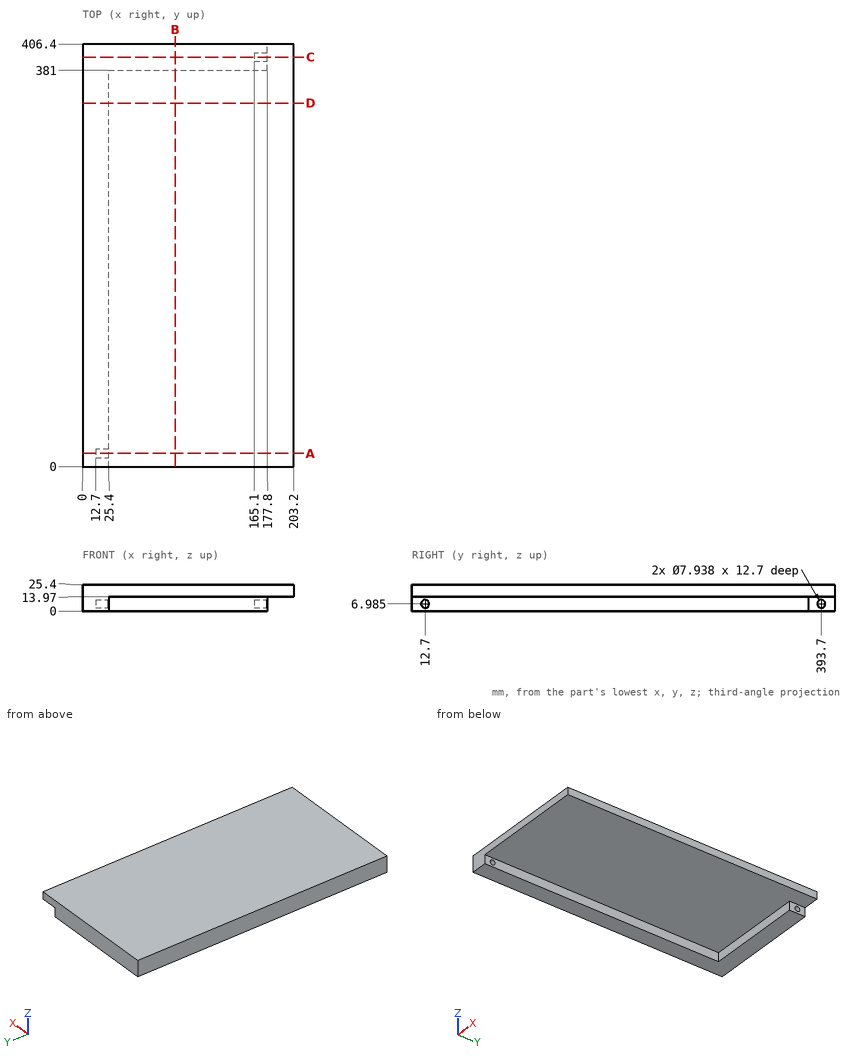
Geometry check sheet. Reference: drawing and pictorial views, mm from the part's lowest x, y, z. Coordinates: 2 decimals unless noted, no trailing zeros. Loops run counter-clockwise (first coordinate to the right, second up) from the corner with the lowest first, then second, coordinate; pieces in that order, holes last. Notation, with made-up numbers: (63, 3) -> (77, 3) arc R15 ccw to (77, 21) -> close; hole circle Ø10 at (12, 87). An arc over 180 degrees is marked (long way). Put each result on its own line as item: value.
1) Cross-section at D-D on y = 349.5. Record the boundary of the cut face in (x, z), plus the area to 3 significant figures.
Result set:
outline: (0, 0) -> (25.4, 0) -> (25.4, 13.97) -> (203.2, 13.97) -> (203.2, 25.4) -> (0, 25.4) -> close
area: 2,680 mm^2
2) Cross-section at A-A on y = 12.7. Record the boundary of the cut face in (x, z), plus the area to 3 significant figures.
Result set:
outline: (0, 0) -> (25.4, 0) -> (25.4, 3.02) -> (12.7, 3.02) -> (12.7, 10.95) -> (25.4, 10.95) -> (25.4, 13.97) -> (203.2, 13.97) -> (203.2, 25.4) -> (0, 25.4) -> close
area: 2,580 mm^2
3) Cross-section at B-B on x = 89. Record the boundary of the cut face in (y, z).
Result set:
outline: (0, 13.97) -> (381, 13.97) -> (381, 0) -> (406.4, 0) -> (406.4, 25.4) -> (0, 25.4) -> close
4) Cross-section at C-C on y = 393.7. Record the boundary of the cut face in (x, z).
Result set:
outline: (0, 0) -> (177.8, 0) -> (177.8, 3.02) -> (165.1, 3.02) -> (165.1, 10.95) -> (177.8, 10.95) -> (177.8, 13.97) -> (203.2, 13.97) -> (203.2, 25.4) -> (0, 25.4) -> close
5) Thickness scan on line 1 (Z direction, x = 19, y = 12.7); line 2 (Z direction, x = 20, y = 12); line 3 (Y direction, x = 99, z = 13). Record the ranges inside material, lowest first.
Result set:
line 1: z = 0 to 3.02, 10.95 to 25.4
line 2: z = 0 to 3.08, 10.89 to 25.4
line 3: y = 381 to 406.4
6) Gauge pin test, flat ends, axial feed: pin 1 Ø2 at (y, z) = (111, 20) entering from -X; pin 2 Ø5 at (x, z) = (30, 7.5) entering from -Y; pin 3 Ø10.5 at (y, z) = (393.7, 6.985) entering from +X; pin 4 Ø1.5 at (x, y) = (82, 258) entering from -Z. Record the tip position at first contact, or that the pin passes through.
Result set:
pin 1: stops at x = 0
pin 2: stops at y = 381
pin 3: stops at x = 177.8
pin 4: stops at z = 13.97
